Verification items for this drawing (mm, ordinates from the low corner). A direction names the side the tool comes from. Round coordinates to 2 decimals unless told otherwise and drop trailing zeros. Write each loop counter-clockwise with the first axis right and the second up, starting at its lowest first coordinate (ties: lowest second). Pieces come first, ordered by that corner, then holes. Notation, with made-up numbers: (81.5, 11.5) -> (140.5, 11.5) arc R21 cw to (140.5, 43.5) -> close; hole circle Ø3 at (11.5, 48). An arc over 180 degrees is marked (long way). One line per item, written item: value.
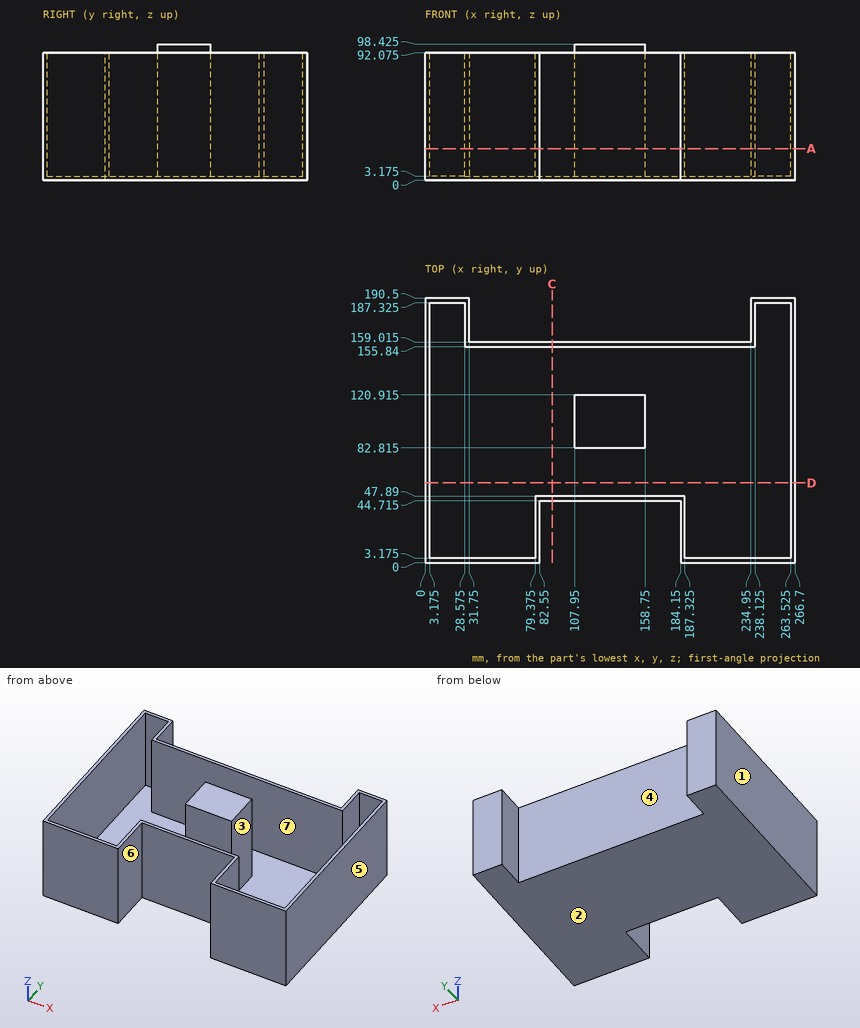
Item 1: Depth check by flat-ended pin: pin 1 (1 mm diameter, centred on x = 57.5, y = 77, fed in from -Z); pin 2 (3 mm diameter, centred on x = 74, y = 156, fed in from +Z) (3 decimals); pin 3 (15 mm diameter, centred on x = 135.5, z = 35.5, fed in from -Y) (1 decimal); pin 4 (10 mm diameter, centred on x = 184.5, z = 26.5, fed in from +Y) (1 decimal). Enter the tip coordinate at first touch or a pass-through.
Result set:
pin 1: z = 0
pin 2: z = 92.075
pin 3: y = 44.7
pin 4: y = 159
Item 2: Sectioned sample at C-C (x = 91.5). Enter the section's corners in (y, z) (1 decimal).
Result set:
outline: (44.7, 0) -> (159, 0) -> (159, 92.1) -> (155.8, 92.1) -> (155.8, 3.2) -> (47.9, 3.2) -> (47.9, 92.1) -> (44.7, 92.1) -> close
Item 3: Material ranges on line 1 along Y through (x, z) = (137, 79) (1 decimal); line 2 along X through (y, z) = (77, 60) (1 decimal); line 3 along Y through (x, z) = (73.5, 10.5) (1 decimal), recorded low to high.
Result set:
line 1: 44.7 to 47.9, 82.8 to 120.9, 155.8 to 159
line 2: 0 to 3.2, 263.5 to 266.7
line 3: 0 to 3.2, 155.8 to 159
Item 4: Sectioned sample at A-A (z = 23). State how many separate pieces and enclosed holes the cut face has, then the cut area to 3 significant figures.
Result set:
separate pieces: 2
enclosed holes: 1
area: 5,280 mm^2
Item 5: Tool access check on the marked faces 4, 5, 6 and 7. Record the directions out of +Z, -Z, +X, -X, +Y, -Y that give a thin tool (end or side, any length) a straight path to the whole face; none if there is none.
Result set:
face 4: +Z, -Z, +Y
face 5: +Z, -Z, +X, +Y, -Y
face 6: +Z, -Z, -Y
face 7: +Z
Item 6: Release check for a two-part mould opening along X. For the marked faces 1, 2 and 3 record: pulls with the +X half, pulls with the -X half, needs draft (parallel to the pull), parting line crosses it, or undercut.
Result set:
face 1: pulls with the -X half
face 2: needs draft
face 3: undercut
Item 7: Sectioned sample at D-D (y = 57.5). Enter the section's corners in (x, z) (1 decimal).
Result set:
outline: (0, 0) -> (266.7, 0) -> (266.7, 92.1) -> (263.5, 92.1) -> (263.5, 3.2) -> (3.2, 3.2) -> (3.2, 92.1) -> (0, 92.1) -> close
